from build123d import *

# Parameters (mm, degrees)
F0_W     = 20
F0_H     = 20
F1_DEPTH = 30
F2_R     = 2.15
F3_DEPTH = 30.001
F4_R     = 2
F5_W     = 3.75
F5_H     = 5.8
F6_DEPTH = 5


with BuildPart() as f1:
    # F0 (on Top) → F1 (new body)
    with BuildSketch(Plane.XY):
        with Locations((10, 10)):
            Rectangle(F0_W, F0_H)
    extrude(amount=F1_DEPTH)

    # F2 (on face) → F3 (cut, through all)
    with BuildSketch(Plane.XY.offset(30)):
        with Locations((10, 10)):
            Circle(F2_R)
    extrude(amount=-F3_DEPTH, mode=Mode.SUBTRACT)

    # F4
    f4_edges = [f1.edges().sort_by_distance(p)[0] for p in [
        (20, 0, 15),
        (0, 0, 15),
        (20, 20, 15),
        (0, 20, 15),
    ]]
    fillet(f4_edges, radius=F4_R)

    # F5 (on face) → F6 (join)
    with BuildSketch(Plane.XY.offset(30)):
        with Locations((1.875, 10)):
            Rectangle(F5_W, F5_H)
        with Locations((18.125, 10)):
            Rectangle(F5_W, F5_H)
    extrude(amount=F6_DEPTH)


solid = f1.part
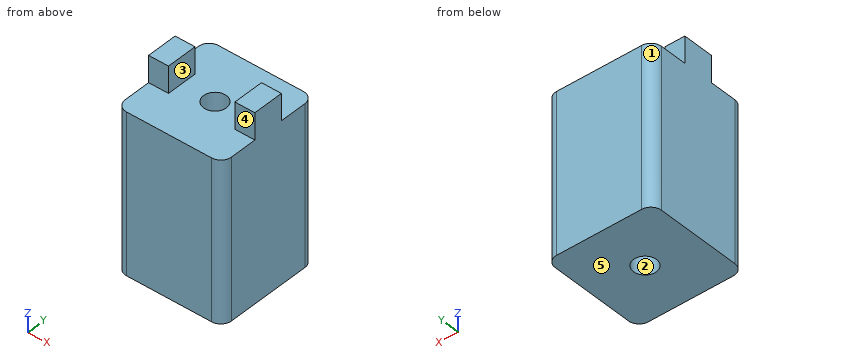
Here's how the part is built. I have some questions about the finished solid (model axes, mm). Face numbers are marked on the shaded views. A direction names the side the tool comes from. Give positions to 0.01 mm unless a question says otherwise; leave off trailing zeros. Order: outer loops, then holes, each group sorted by start corner. A loop starts at its lowest first (then second) coordinate and runs counter-clockwise, first axis right, second up. Notation, with made-up numbers: M 31,54 L 56,54 A23 cw 56,69 Z; hole C 87.5,17.5 d6. An arc over 180 degrees is marked long. Answer as a JSON object with one key per item and string values. Group by question number.
1) We'd pull the mould along Y, two halves only. Please class the marked faces 1, 2 and 3: pulls with the +Y half, pulls with the -Y half, needs draft (parallel to the pull), parting line crosses it, or undercut.
2) On a 3-axis mill with a long thin cutter (end or side, diameter ignored), from which of +Z, -Z, +X, -X, +Y, -Y can I reach the whole of each face in a straight line? I mean the marked faces 4 and 5. Say none if no direction works.
3) Suppose I cut it at B-B, the plane x = 10. Write out the boundary of the cut face in (y, z), plus the area to 3 significant figures.
4) I'm going to push flat-ended pins straight in: pin 1 Ø4 at (x, z) = (1.5, 32.5) entering from +Y; pin 2 Ø4 at (y, z) = (9, 33.5) entering from -X; pin 3 Ø1.9 at (x, z) = (17.5, 32) entering from -Y; pin 4 Ø6 at (x, y) = (12, 7) entering from +Z. Where does each tip first touch, or does it pass through?
5) Please list where these lines run through material, in increasing order: L1, parallel to X at y = 12.25, z = 32.5; L2, parallel to Y at x = 10, z = 11.25; L3, parallel to Z at x = 15, y = 18. Write a range as [from, to].
6) Suppose I cut it at D-D, the plane x = 17. Write out the boundary of the cut face in (y, z).
7) Suppose I cut it at A-A, the plane y = 10. Write out the boundary of the cut face in (x, z).
8) Suppose I cut it at C-C, the plane z = 29. Write out the boundary of the cut face in (x, y), plus the area to 3 significant figures.
Results found:
{
 "1": {"face 1": "pulls with the +Y half", "face 2": "undercut", "face 3": "needs draft"},
 "2": {"face 4": "+Z, +X, -X, -Y", "face 5": "-Z, +X, -X, +Y, -Y"},
 "3": {"outline": "M 0,0 L 7.85,0 L 7.85,30 L 0,30 Z; M 12.15,0 L 20,0 L 20,30 L 12.15,30 Z", "area": "471 mm²"},
 "4": {"pin 1": "y = 12.9", "pin 2": "x = 0", "pin 3": "y = 7.1", "pin 4": "z = 30"},
 "5": {"L1": "[0, 3.75], [16.25, 20]", "L2": "[0, 7.85], [12.15, 20]", "L3": "[0, 30]"},
 "6": {"outline": "M 0,0 L 20,0 L 20,30 L 12.9,30 L 12.9,35 L 7.1,35 L 7.1,30 L 0,30 Z"},
 "7": {"outline": "M 0,0 L 7.85,0 L 7.85,30 L 3.75,30 L 3.75,35 L 0,35 Z; M 12.15,0 L 20,0 L 20,35 L 16.25,35 L 16.25,30 L 12.15,30 Z"},
 "8": {"outline": "M 0,2 A2 ccw 2,0 L 18,0 A2 ccw 20,2 L 20,18 A2 ccw 18,20 L 2,20 A2 ccw 0,18 Z; hole C 10,10 d4.3", "area": "382 mm²"}
}
